Input: part model. Units: mm. Frame: model coordinates. Face numbers are marked on the shaded views. A direction names the side the tool comes from. Coordinates: 2 decimals unless noted, no trailing zeros. Write each loop counter-clockwise with the first axis right and the second up, starting at its lowest first coordinate (ties: lowest second). Pieces come first, ordered by that corner, then holes. Notation, with made-up numbers: M -21.75,57.5 L -3.75,57.5 A9 ccw -3.75,70.5 Z; hole C 12,28.25 d11. An arc over 180 degrees is marked long. Write each question's results on one line, items separated by ' | '. Start each with the question number.
1. Ray query, probe 1 along Y at (x, z) = (9.25, 12.9); probe 2 along Z at (x, y) = (7.5, 3.75); probe 3 along Z at (x, y) = (16, 4). Return the intervals inside material, ascending.
2. Section query B-B, the plane z = -0.75. Output: boundary loops of the cut face in (x, y), and give its area (3 significant figures).
3. First-contact query: pin 1 (1 mm diameter, centred on y = 11.5, z = 4, fed in from +X); pin 2 (4 mm diameter, centred on x = 8, y = 8.5, fed in from +Z); pin 3 (2 mm diameter, centred on x = 20.5, y = 10.5, fed in from -Z). Flat tips, straight axial feed; report the tip coordinate or a pass-through.
4. Set-up query: the marked faces 4, 5 and 6. Return all of +Z, -Z, +X, -X, +Y, -Y with unobstructed straight access to the full face (end or side cutting, diameter ignored); none if empty.
5. Pull-direction query (Y, two-part tool) for the marked faces 1, 2 and 3; classes: +Y half, -Y half, draft (parallel to the pull), parting line (faces both ways), or undercut.
6. Section query A-A, the plane y = -2. Output: boundary loops of the cut face in (x, z).
7. Section query C-C, the plane x = 9.25. Output: boundary loops of the cut face in (y, z), and give its area (3 significant figures).
8. Section query D-D, the plane y = 6.25. Output: boundary loops of the cut face in (x, z).
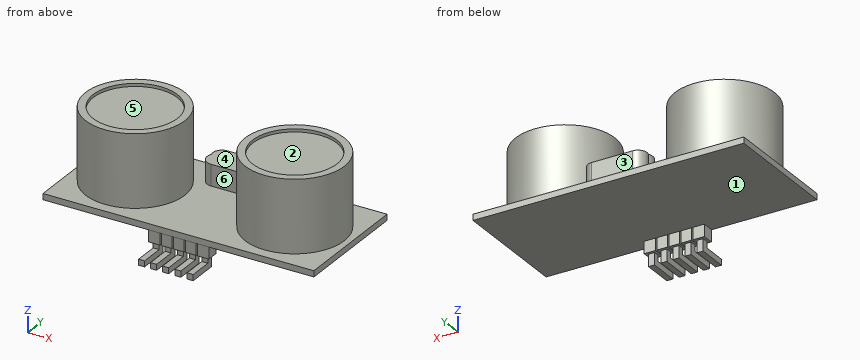
```python
from build123d import *

# Parameters (mm, degrees)
ESBO_O1_W                = 45
ESBO_O1_H                = 20
RESSALTO_EXTRUS_O1_DEPTH = 1
ESBO_O2_R                = 8.25
RESSALTO_EXTRUS_O2_DEPTH = 12
ESBO_O3_R                = 7
CORTE_EXTRUS_O1_DEPTH    = 0.5
RESSALTO_EXTRUS_O5_DEPTH = 3.5
ESBO_O7_W                = 1.9
ESBO_O7_H                = 2
ESBO_O7_W_2              = 1.8
RESSALTO_EXTRUS_O6_DEPTH = 2
ESBO_O9_W                = 10
ESBO_O9_H                = 0.1
CORTE_EXTRUS_O2_DEPTH    = 2
ESBO_O10_W               = 1
ESBO_O10_H               = 1
RESSALTO_EXTRUS_O7_DEPTH = 2
ESBO_O11_W               = 1
ESBO_O11_H               = 1
ESBO_O11_H_2             = 0.967747288
RESSALTO_EXTRUS_O8_DEPTH = 4
RESSALTO_EXTRUS_O3_DEPTH = 3.5


with BuildPart() as part:
    # Esboço1 → Ressalto-extrusão1 (new body)
    with BuildSketch(Plane.XY):
        with Locations((22.5, 10)):
            Rectangle(ESBO_O1_W, ESBO_O1_H)
    extrude(amount=RESSALTO_EXTRUS_O1_DEPTH)

    # Esboço2 → Ressalto-extrusão2 (add)
    with BuildSketch(Plane.XY.offset(1)):
        with Locations((9.25, 10)):
            Circle(ESBO_O2_R)
        with Locations((35.75, 10)):
            Circle(ESBO_O2_R)
    extrude(amount=RESSALTO_EXTRUS_O2_DEPTH)

    # Esboço3 → Corte-extrusão1 (cut)
    with BuildSketch(Plane.XY.offset(13)):
        with Locations((9.25, 10)):
            Circle(ESBO_O3_R)
        with Locations((35.75, 10)):
            Circle(ESBO_O3_R)
    extrude(amount=-CORTE_EXTRUS_O1_DEPTH, mode=Mode.SUBTRACT)

    # Esboço6 → Ressalto-extrusão5 (add)
    with BuildSketch(Plane.XY.offset(1)):
        with BuildLine():
            Line((25.75, 17.816758405), (19.25, 17.816758405))
            ThreePointArc((19.25, 17.816758405), (17.5, 16.066758405), (19.25, 14.316758405))
            Line((19.25, 14.316758405), (25.75, 14.316758405))
            ThreePointArc((25.75, 14.316758405), (27.5, 16.066758405), (25.75, 17.816758405))
        make_face()
    extrude(amount=RESSALTO_EXTRUS_O5_DEPTH)

    # Esboço7 → Ressalto-extrusão6 (add)
    with BuildSketch(Plane(origin=(0, 0, 0), x_dir=(-1, 0, 0), z_dir=(0, 0, -1))):
        with Locations((-26.55, 1)):
            Rectangle(ESBO_O7_W, ESBO_O7_H)
        with Locations((-24.5, 1)):
            Rectangle(ESBO_O7_W_2, ESBO_O7_H)
        with Locations((-22.5, 1)):
            Rectangle(ESBO_O7_W_2, ESBO_O7_H)
        with Locations((-20.5, 1)):
            Rectangle(ESBO_O7_W_2, ESBO_O7_H)
        with Locations((-18.45, 1)):
            Rectangle(ESBO_O7_W, ESBO_O7_H)
    extrude(amount=RESSALTO_EXTRUS_O6_DEPTH)

    # Esboço9 → Corte-extrusão2 (cut)
    with BuildSketch(Plane(origin=(0, 0, -2), x_dir=(-1, 0, 0), z_dir=(0, 0, -1))):
        with Locations((-22.5, 0.05)):
            Rectangle(ESBO_O9_W, ESBO_O9_H)
    extrude(amount=-CORTE_EXTRUS_O2_DEPTH, mode=Mode.SUBTRACT)

    # Esboço10 → Ressalto-extrusão7 (add)
    with BuildSketch(Plane(origin=(0, 0, -2), x_dir=(-1, 0, 0), z_dir=(0, 0, -1))):
        with Locations((-24.5, 1.05)):
            Rectangle(ESBO_O10_W, ESBO_O10_H)
        with Locations((-26.55, 1.05)):
            Rectangle(ESBO_O10_W, ESBO_O10_H)
        with Locations((-22.472435469, 1.05)):
            Rectangle(ESBO_O10_W, ESBO_O10_H)
        with Locations((-20.46939422, 1.05)):
            Rectangle(ESBO_O10_W, ESBO_O10_H)
        with Locations((-18.471440092, 1.05)):
            Rectangle(ESBO_O10_W, ESBO_O10_H)
    extrude(amount=RESSALTO_EXTRUS_O7_DEPTH)

    # Esboço11 → Ressalto-extrusão8 (add)
    with BuildSketch(Plane.XZ.offset(-0.55)):
        with Locations((26.55, -3.5)):
            Rectangle(ESBO_O11_W, ESBO_O11_H)
        with Locations((24.5, -3.5)):
            Rectangle(ESBO_O11_W, ESBO_O11_H)
        with Locations((22.472435469, -3.516126356)):
            Rectangle(ESBO_O11_W, ESBO_O11_H_2)
        with Locations((20.46939422, -3.516126356)):
            Rectangle(ESBO_O11_W, ESBO_O11_H_2)
        with Locations((18.471440092, -3.516126356)):
            Rectangle(ESBO_O11_W, ESBO_O11_H_2)
    extrude(amount=RESSALTO_EXTRUS_O8_DEPTH)

    # Esboço4 → Ressalto-extrusão3 (add)
    with BuildSketch(Plane.XY.offset(1)):
        with BuildLine():
            ThreePointArc((20.566173289, 17.816758405), (20.042035666, 18.667291225), (19.1, 19))
            ThreePointArc((19.1, 19), (17.849334275, 18.328151704), (17.719012065, 16.914446994))
            ThreePointArc((17.719012065, 16.914446994), (18.361449222, 17.574398122), (19.25, 17.816758405))
            Line((19.25, 17.816758405), (20.566173289, 17.816758405))
        make_face()
        with BuildLine():
            ThreePointArc((20.6, 17.5), (20.591519348, 17.659279733), (20.566173289, 17.816758405))
            Line((20.566173289, 17.816758405), (19.25, 17.816758405))
            ThreePointArc((19.25, 17.816758405), (18.361449222, 17.574398122), (17.719012065, 16.914446994))
            ThreePointArc((17.719012065, 16.914446994), (18.271848296, 16.249334275), (19.1, 16))
            ThreePointArc((19.1, 16), (20.160660172, 16.439339828), (20.6, 17.5))
        make_face()
        with BuildLine():
            Line((25.9, 19), (19.1, 19))
            ThreePointArc((19.1, 19), (20.042035666, 18.667291225), (20.566173289, 17.816758405))
            Line((20.566173289, 17.816758405), (24.433826711, 17.816758405))
            ThreePointArc((24.433826711, 17.816758405), (24.957964334, 18.667291225), (25.9, 19))
        make_face()
        with BuildLine():
            ThreePointArc((27.4, 17.5), (26.960660172, 18.560660172), (25.9, 19))
            ThreePointArc((25.9, 19), (24.957964334, 18.667291225), (24.433826711, 17.816758405))
            Line((24.433826711, 17.816758405), (25.75, 17.816758405))
            ThreePointArc((25.75, 17.816758405), (26.638550778, 17.574398122), (27.280987935, 16.914446994))
            ThreePointArc((27.280987935, 16.914446994), (27.369945901, 17.201237471), (27.4, 17.5))
        make_face()
        with BuildLine():
            Line((25.75, 17.816758405), (24.433826711, 17.816758405))
            ThreePointArc((24.433826711, 17.816758405), (24.732708775, 16.557964334), (25.9, 16))
            ThreePointArc((25.9, 16), (26.728151704, 16.249334275), (27.280987935, 16.914446994))
            ThreePointArc((27.280987935, 16.914446994), (26.638550778, 17.574398122), (25.75, 17.816758405))
        make_face()
        with BuildLine():
            Line((24.433826711, 17.816758405), (20.566173289, 17.816758405))
            ThreePointArc((20.566173289, 17.816758405), (20.591519348, 17.659279733), (20.6, 17.5))
            ThreePointArc((20.6, 17.5), (20.160660172, 16.439339828), (19.1, 16))
            Line((19.1, 16), (25.9, 16))
            ThreePointArc((25.9, 16), (24.732708775, 16.557964334), (24.433826711, 17.816758405))
        make_face()
    extrude(amount=RESSALTO_EXTRUS_O3_DEPTH)


solid = part.part
```
Answer:
1) probe 1: 1.75 to 3, 17 to 18.25 | probe 2: 0 to 12.5 | probe 3: 0 to 1
2) outline: M 17.5,0.1 L 19.4,0.1 L 19.4,2 L 17.5,2 Z; M 19.6,0.1 L 21.4,0.1 L 21.4,2 L 19.6,2 Z; M 21.6,0.1 L 23.4,0.1 L 23.4,2 L 21.6,2 Z; M 23.6,0.1 L 25.4,0.1 L 25.4,2 L 23.6,2 Z; M 25.6,0.1 L 27.5,0.1 L 27.5,2 L 25.6,2 Z | area: 17.5 mm^2
3) pin 1: x = 43.94 | pin 2: z = 12.5 | pin 3: z = 0
4) face 4: +Z, +Y, -Y | face 5: +Z | face 6: +Z, -Y
5) face 1: draft | face 2: undercut | face 3: +Y half
6) outline: M 17.97,-4 L 18.97,-4 L 18.97,-3.03 L 17.97,-3.03 Z; M 19.97,-4 L 20.97,-4 L 20.97,-3.03 L 19.97,-3.03 Z; M 21.97,-4 L 22.97,-4 L 22.97,-3.03 L 21.97,-3.03 Z; M 24,-4 L 25,-4 L 25,-3 L 24,-3 Z; M 26.05,-4 L 27.05,-4 L 27.05,-3 L 26.05,-3 Z
7) outline: M 0,0 L 20,0 L 20,1 L 18.25,1 L 18.25,13 L 17,13 L 17,12.5 L 3,12.5 L 3,13 L 1.75,13 L 1.75,1 L 0,1 Z | area: 211 mm^2
8) outline: M 0,0 L 45,0 L 45,1 L 43.1,1 L 43.1,13 L 41.66,13 L 41.66,12.5 L 29.84,12.5 L 29.84,13 L 28.4,13 L 28.4,1 L 16.6,1 L 16.6,13 L 15.16,13 L 15.16,12.5 L 3.34,12.5 L 3.34,13 L 1.9,13 L 1.9,1 L 0,1 Z
